from build123d import *

# Parameters (mm, degrees)
F0_W     = 399.9802543244
F0_H     = 609.6
F1_DEPTH = 53.34
F2_W     = 78.0126031023
F2_H     = 133.5061052814
F3_DEPTH = 52.07
F4_W     = 133.5061052814
F4_H     = 51.0229802537
F5_DEPTH = 10.16
F6_R     = 1.8396087238
F6_R_2   = 1.9116150916
F7_DEPTH = 25.4


with BuildPart() as f1:
    # F0 (on Top) → F1 (new body)
    with BuildSketch(Plane.XY):
        with Locations((199.9901271622, 304.8)):
            Rectangle(F0_W, F0_H)
    extrude(amount=F1_DEPTH)

    # F2 (on face) → F3 (cut)
    with BuildSketch(Plane.XY.offset(53.34)):
        with Locations((42.3716591904, 71.9645838253)):
            Rectangle(F2_W, F2_H)
    extrude(amount=-F3_DEPTH, mode=Mode.SUBTRACT)

    # F4 (on face) → F5 (cut)
    with BuildSketch(Plane(origin=(81.3779607415, 0, 0), x_dir=(0, -1, 0), z_dir=(-1, 0, 0))):
        with Locations((-71.9645838253, 26.7814901268)):
            Rectangle(F4_W, F4_H)
    extrude(amount=-F5_DEPTH, mode=Mode.SUBTRACT)

    # F6 (on face) → F7 (cut)
    with BuildSketch(Plane.XY.offset(53.34)):
        with Locations((86.4754936327, 130.9549957514)):
            Circle(F6_R)
        with BuildLine():
            Line((84.4225700873, 121.4809922279), (84.4225700873, 117.0233345083))
            ThreePointArc((84.4225700873, 117.0233345083), (86.1374283625, 114.22337587), (88.6342981207, 116.3555458188))
            Line((88.6342981207, 116.3555458188), (88.6336831498, 116.4070708193))
            Line((88.6336831498, 116.4070708193), (88.5679829552, 121.9117257152))
            ThreePointArc((88.5679829552, 121.9117257152), (86.6669107252, 123.970616392), (84.4225700873, 122.2925098566))
            Line((84.4225700873, 122.2925098566), (84.4225700873, 121.4809922279))
        make_face()
        with Locations((86.4754936327, 110.0129559636)):
            Circle(F6_R_2)
    extrude(amount=-F7_DEPTH, mode=Mode.SUBTRACT)


solid = f1.part
Can you work these out from the model? Positions are in its coordinate system, mm. Coordinates: 2 decimals unless noted, no trailing zeros. Write each loop counter-clockwise with the first axis right and the second up, starting at its lowest first coordinate (ties: lowest second). Pieces come first, ordered by that corner, then holes. Notation, with made-up numbers: M -17,5 L 24,5 A17 ccw 24,10 Z; hole C -4,76.25 d11. An arc over 180 degrees is marked long. Use one line per item in the form item = value.
Q1. I need wall thicknesses on line 1 along X through (y, z) = (126, 10.5); line 2 along Y through (x, z) = (70.5, 32.5); line 3 along Z through (x, y) = (63, 81.5). Which ranges of each line are inside material? Lowest first, please. Write a range as from..to.
Model answer:
line_1 = 0..3.37, 91.54..399.98
line_2 = 0..5.21, 138.72..609.6
line_3 = 0..1.27
Q2. If we section it at A-A (z = 34.5): Write out the boundary of the cut face in (x, y).
Model answer:
outline = M 0,0 L 399.98,0 L 399.98,609.6 L 0,609.6 Z; hole M 3.37,5.21 L 91.54,5.21 L 91.54,138.72 L 3.37,138.72 Z
Q3. We'd pull the mould along X, two halves only. Please class faces 1 (the flat face through (197, 309, 53.34)), 2 (the flat face through (399.98, 301, 26)), 3 (the flat face through (3.365, 71, 28)), 4 (the flat face through (91.538, 73, 27)): +X half, -X half, draft (parallel to the pull), parting line (faces both ways), or undercut.
Model answer:
face_1 = draft
face_2 = +X half
face_3 = undercut
face_4 = undercut
Q4. If we section it at B-B (y = 89): Write out the boundary of the cut face in (x, z).
Model answer:
outline = M 0,0 L 399.98,0 L 399.98,53.34 L 81.38,53.34 L 81.38,52.29 L 91.54,52.29 L 91.54,1.27 L 3.37,1.27 L 3.37,53.34 L 0,53.34 Z
